Geometry check sheet. Reference: the model listing, model coordinates, mm. Face numbers are marked on the shaded views. A direction names the side the tool comes from. Round coordinates to 2 decimals unless told otherwise and drop trailing zeros. Loops run counter-clockwise (first coordinate to the right, second up) from the corner with the lowest first, then second, coordinate; pieces in that order, holes last. Notation, with made-up numbers: (81, 20) -> (132, 20) arc R13 cw to (132, 36) -> close; hole circle Ø11 at (77.5, -29.5). An arc over 180 degrees is marked (long way). Use one line per item in the form item = value.
from build123d import *

# Parameters (mm, degrees)
EXTRUDE_2_DEPTH     = 6.5
SKETCH_3_R          = 10
EXTRUDE_3_DEPTH     = 2
EXTRUDE_START       = 2
SKETCH_4_R          = 10
EXTRUDE_4_DEPTH     = 2
SKETCH_5_R          = 5
EXTRUDE_5_DEPTH     = 1.5
SKETCH_8_W          = 6
SKETCH_8_H          = 6.5
CUT_EXTRUDE_2_DEPTH = 0.94
SKETCH_9_W          = 6
SKETCH_9_H          = 6.5
CUT_EXTRUDE_3_DEPTH = 0.94
FILLET_4_R          = 2
SKETCH_10_W         = 15
SKETCH_10_H         = 2.5
EXTRUDE_6_DEPTH     = 6.8
SKETCH_11_W         = 15
SKETCH_11_H         = 18
SKETCH_11_H_2       = 6.5
EXTRUDE_7_DEPTH     = 6.8
SKETCH_12_W         = 15
SKETCH_12_H         = 7
EXTRUDE_8_DEPTH     = 13.2
SKETCH_16_W         = 15
SKETCH_16_H         = 18
SKETCH_16_H_2       = 2.5
EXTRUDE_10_DEPTH    = 3
SKETCH_17_W         = 15
SKETCH_17_H         = 20
CUT_EXTRUDE_6_DEPTH = 3
SKETCH_18_W         = 15
SKETCH_18_H         = 7
CUT_EXTRUDE_7_DEPTH = 3
FILLET_7_R          = 8


with BuildPart() as part:
    # Sketch 1 → Extrude 2 (new body)
    with BuildSketch(Plane(origin=(0, 0, 0), x_dir=(1, 0, 0), z_dir=(0, 1, 0))):
        with BuildLine():
            Line((-9.5, 0), (-9.5, -7.5))
            Line((-9.5, -7.5), (-8.44, -7.5))
            Line((-8.44, -7.5), (-8.44, -13.5))
            Line((-8.44, -13.5), (8.44, -13.5))
            Line((8.44, -13.5), (8.44, -7.5))
            Line((8.44, -7.5), (9.5, -7.5))
            Line((9.5, -7.5), (9.5, 0))
            ThreePointArc((9.5, 0), (0, 9.438928409), (-9.5, 0))
        make_face()
    extrude(amount=EXTRUDE_2_DEPTH)

    # Sketch 3 → Extrude 3 (add)
    with BuildSketch(Plane(origin=(0, 6.5, 0), x_dir=(1, 0, 0), z_dir=(0, 1, 0))):
        with Locations(Location((0, 0, 0), (0, 0, 198.194872339))):
            Circle(SKETCH_3_R)
    extrude(amount=EXTRUDE_3_DEPTH)

    # Sketch 4 → Extrude 4 (add)
    with BuildSketch(Plane.XZ.offset(EXTRUDE_START)):
        with Locations(Location((0, 0, 0), (0, 0, 161.805127661))):
            Circle(SKETCH_4_R)
    extrude(amount=-EXTRUDE_4_DEPTH)

    # Sketch 5 → Extrude 5 (add)
    with BuildSketch(Plane.XZ.offset(2)):
        with Locations(Location((0, 0, 0), (0, 0, 270))):
            Circle(SKETCH_5_R)
    extrude(amount=EXTRUDE_5_DEPTH)

    # Sketch 8 → Cut-Extrude 2 (cut)
    with BuildSketch(Plane(origin=(8.44, 0, 0), x_dir=(0, 0, -1), z_dir=(1, 0, 0))):
        with Locations((-10.5, 3.25)):
            Rectangle(SKETCH_8_W, SKETCH_8_H)
    extrude(amount=-CUT_EXTRUDE_2_DEPTH, mode=Mode.SUBTRACT)

    # Sketch 9 → Cut-Extrude 3 (cut)
    with BuildSketch(Plane.ZY.offset(8.44)):
        with Locations((10.5, 3.25)):
            Rectangle(SKETCH_9_W, SKETCH_9_H)
    extrude(amount=-CUT_EXTRUDE_3_DEPTH, mode=Mode.SUBTRACT)

    # Fillet 4
    fillet_4_edges = [part.edges().sort_by_distance(p)[0] for p in [
        (7.5, 3.25, 7.5),
        (-7.5, 3.25, 7.5),
    ]]
    fillet(fillet_4_edges, radius=FILLET_4_R - 0.0001)  # a hair under: the kernel refuses the full size



with BuildPart() as body_2:
    # Sketch 10 → Extrude 6 (new body)
    with BuildSketch(Plane.XY.offset(13.5)):
        with Locations((0, -1.25)):
            Rectangle(SKETCH_10_W, SKETCH_10_H)
    extrude(amount=EXTRUDE_6_DEPTH)


with BuildPart() as part_1:
    add(part.part)

    add(body_2.part)  # Extrude 7 merges body 2
    # Sketch 11 → Extrude 7 (add)
    with BuildSketch(Plane.XY.offset(13.5)):
        with Locations((0, 15.5)):
            Rectangle(SKETCH_11_W, SKETCH_11_H)
        with Locations((0, 3.25)):
            Rectangle(SKETCH_11_W, SKETCH_11_H_2)
    extrude(amount=EXTRUDE_7_DEPTH)

    # Sketch 12 → Extrude 8 (add)
    with BuildSketch(Plane.XY.offset(20.3)):
        with Locations((0, 21)):
            Rectangle(SKETCH_12_W, SKETCH_12_H)
    extrude(amount=EXTRUDE_8_DEPTH)

    # Sketch 16 → Extrude 10 (add)
    with BuildSketch(Plane(origin=(0, 0, 13.5), x_dir=(-1, 0, 0), z_dir=(0, 0, -1))):
        with Locations((0, 15.5)):
            Rectangle(SKETCH_16_W, SKETCH_16_H)
        with Locations((0, -1.25)):
            Rectangle(SKETCH_16_W, SKETCH_16_H_2)
    extrude(amount=EXTRUDE_10_DEPTH)

    # Sketch 17 → Cut-Extrude 6 (cut)
    with BuildSketch(Plane.XY.offset(20.3)):
        with Locations((0, 7.5)):
            Rectangle(SKETCH_17_W, SKETCH_17_H)
    extrude(amount=-CUT_EXTRUDE_6_DEPTH, mode=Mode.SUBTRACT)

    # Sketch 18 → Cut-Extrude 7 (cut)
    with BuildSketch(Plane.XY.offset(33.5)):
        with Locations((0, 21)):
            Rectangle(SKETCH_18_W, SKETCH_18_H)
    extrude(amount=-CUT_EXTRUDE_7_DEPTH, mode=Mode.SUBTRACT)

    # Fillet 7
    fillet_7_edges = [part_1.edges().sort_by_distance(p)[0] for p in [
        (0, 17.5, 17.3),
    ]]
    fillet(fillet_7_edges, radius=FILLET_7_R)


solid = part_1.part
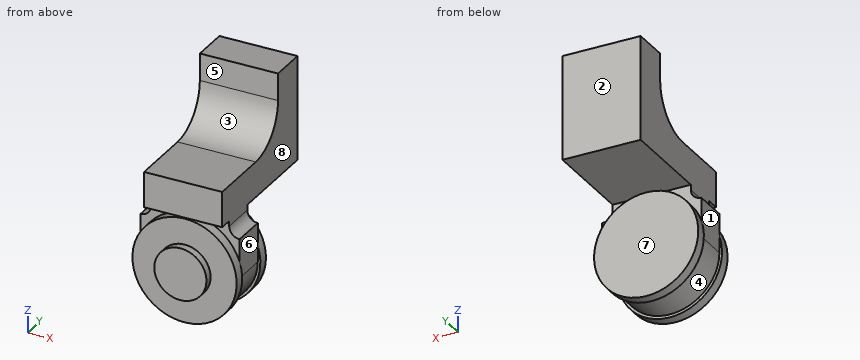
1. Section check A-A (x = 0). Record the boundary of the cut face in (y, z), then the cut area to 3 significant figures.
Return value:
outline = (-3.5, -5) -> (-2, -5) -> (-2, -10) -> (0, -10) -> (0, -9.44) -> (6.5, -9.44) -> (6.5, -10) -> (8.5, -10) -> (8.5, 10) -> (6.5, 10) -> (6.5, 10.5) -> (24.5, 10.5) -> (24.5, 30.5) -> (17.5, 30.5) -> (17.5, 25.3) arc R8 cw to (9.5, 17.3) -> (-2.5, 17.3) -> (-2.5, 10.5) -> (0, 10.5) -> (0, 10) -> (-2, 10) -> (-2, 5) -> (-3.5, 5) -> close
area = 514 mm2
2. Mould release check, pull along Y, two halves, no side actions. Record for the marked faces 1, 2 and 3: released by +Y, released by -Y, zero draft, split by the parting line, or undercut.
Return value:
face_1 = undercut
face_2 = released by +Y
face_3 = released by -Y
3. Material ranges on line 1 along Y through (x, z) = (6.5, -7.5); line 2 along Y through (x, z) = (-3, 5.5); line 3 along Z through (x, y) = (-2.5, 19), recorded low to high.
Return value:
line_1 = -2 to 0, 6.5 to 8.5
line_2 = -2 to 8.5
line_3 = 10.5 to 30.5
4. Section check D-D (y = 17). Record the boundary of the cut face in (x, z), then the cut area to 3 significant figures.
Return value:
outline = (-7.5, 10.5) -> (7.5, 10.5) -> (7.5, 22.52) -> (-7.5, 22.52) -> close
area = 180 mm2
5. Gauge pin test, flat ends, axial feed: pin 1 (5 mm diameter, centred on x = 3, z = 2, fed in from +Y); pin 2 (7.5 mm diameter, centred on x = 3.5, z = 15, fed in from -Y); pin 3 (5 mm diameter, centred on x = 7.5, z = 7.5, fed in from -Y). Record the tip position at first contact, or that the pin passes through.
Return value:
pin_1 = 8.5
pin_2 = -2.5
pin_3 = -2
6. Section check B-B (z = -6). Record the boundary of the cut face in (x, y), then the cut area to 3 significant figures.
Return value:
outline = (-8, -2) -> (8, -2) -> (8, 0) -> (7.32, 0) -> (7.32, 6.5) -> (8, 6.5) -> (8, 8.5) -> (-8, 8.5) -> (-8, 6.5) -> (-7.32, 6.5) -> (-7.32, 0) -> (-8, 0) -> close
area = 159 mm2
7. Tool access check on the marked faces 4, 5, 6, 7 and 8. Record the directions out of +Z, -Z, +X, -X, +Y, -Y that give a thin tool (end or side, any length) a straight path to the whole face; none if there is none.
Return value:
face_4 = -Z
face_5 = +Z, +X, -X, -Y
face_6 = +Z, -Z, +X
face_7 = -Z, +X, -X, +Y
face_8 = +Z, +X, +Y, -Y
8. Section check C-C (x = -6.25). Record the boundary of the cut face in (y, z).
Return value:
outline = (-2.5, 10.5) -> (0, 10.5) -> (0, 7.81) -> (-2, 7.81) -> (-2, -7.81) -> (0, -7.81) -> (0, -7.09) -> (6.5, -7.09) -> (6.5, -7.81) -> (8.5, -7.81) -> (8.5, 7.81) -> (6.5, 7.81) -> (6.5, 10.5) -> (24.5, 10.5) -> (24.5, 30.5) -> (17.5, 30.5) -> (17.5, 25.3) arc R8 cw to (9.5, 17.3) -> (-2.5, 17.3) -> close
